Autodesk Inventor part; units mm, degrees
ref_plane "YZ Plane" through (0, 0, 0) normal (1, 0, 0) x (0, 1, 0)
ref_plane "XZ Plane" through (0, 0, 0) normal (0, 1, 0) x (-1, 0, 0)
ref_plane "XY Plane" through (0, 0, 0) normal (0, 0, 1) x (1, 0, 0)
sketch "スケッチ1" plane through (0, 0, 0) normal (0, 0, 1) x (1, 0, 0)
  line L0 (0, 0) -> (80, 0)
  line L1 (80, 0) -> (80, 60)
  line L2 (80, 60) -> (0, 60)
  line L3 (0, 60) -> (0, 0)
  dimension "d0" = 80
  dimension "d1" = 60
extrude "押し出し1" add sketch "スケッチ1" along normal blind 3
sketch "スケッチ2" plane through (0, 0, 3) normal (0, 0, 1) x (1, 0, 0)
  point P0 (0, 0)
sketch "スケッチ3" plane through (0, 0, 3) normal (0, 0, 1) x (1, 0, 0)
  line L0 (0, 0) -> (80, 0)
  line L1 (15, 0) -> (15, 60) construction
  line L2 (15, 0) -> (75, 0) construction
  line L3 (0, 60) -> (0, 0)
  circle A0 centre (7.5, 30) radius 1.6
  circle A1 centre (7.5, 40) radius 1.6
  circle A2 centre (7.5, 20) radius 1.6
  line L4 (80, 60) -> (0, 60)
  line L5 (40, 60) -> (40, 0) construction
  circle A3 centre (72.5, 30) radius 1.6
  circle A4 centre (72.5, 40) radius 1.6
  circle A5 centre (72.5, 20) radius 1.6
  point P0 (0, 30)
  dimension "d4" = 60
  dimension "d5" = 90
  dimension "d6" = 15
  dimension "d7" = 3.2
  dimension "d8" = 7.5
  dimension "d9" = 30
  dimension "d10" = 3.2
  dimension "d11" = 3.2
  dimension "d12" = 10
  dimension "d13" = 10
  dimension "d14" = 40
hole "穴1" at (7.5, 40, 3) at (7.5, 30, 3) at (7.5, 20, 3) at (72.5, 40, 3) at (72.5, 30, 3) at (72.5, 20, 3) direction (0, 0, -1) diameter 3.2 end through all
sketch "スケッチ4" plane through (0, 0, 3) normal (0, 0, 1) x (1, 0, 0)
  circle A0 centre (40, 30) radius 7.5
  line L0 (80, 60) -> (0, 60)
  line L1 (80, 0) -> (80, 60)
  point P0 (0, 0)
  dimension "d22" = 15
  dimension "d23" = 30
  dimension "d24" = 40
extrude "押し出し2" cut sketch "スケッチ4" against normal blind 3
sketch "スケッチ5" plane through (0, 0, 3) normal (0, 0, 1) x (1, 0, 0)
  point P0 (0, 0)
sketch "スケッチ6" plane through (0, 0, 3) normal (0, 0, 1) x (1, 0, 0)
  circle A0 centre (40, 30) radius 7.5
  circle A1 centre (40, 30) radius 12.05
  point P0 (0, 0)
  dimension "d27" = 24.1
extrude "押し出し3" cut sketch "スケッチ6" against normal blind 3
sketch "スケッチ7" plane through (0, 0, 3) normal (0, 0, 1) x (1, 0, 0)
  circle A0 centre (40, 30) radius 12.05
  line L0 (0, 0) -> (80, 0)
  point P0 (62.851, 30)
  point P1 (17.149, 30)
  dimension "d30" = 22.851
  dimension "d31" = 22.851
  dimension "d32" = 30
  dimension "d33" = 30
hole "穴2" at (17.149, 30, 3) at (62.851, 30, 3) direction (0, 0, -1) diameter 3.2 end through all
fillet "フィレット1" radius 6 4 edges at (0, 60, 1.5) (80, 60, 1.5) (80, 0, 1.5) (0, 0, 1.5)
sketch "スケッチ8" plane through (0, 0, 3) normal (0, 0, 1) x (1, 0, 0)
  point P0 (0, 0)
sketch "スケッチ9" plane through (0, 0, 3) normal (0, 0, 1) x (1, 0, 0)
  circle A0 centre (40, 30) radius 12.05
  circle A1 centre (40, 30) radius 9.6
  point P0 (0, 0)
  dimension "d42" = 19.2
extrude "押し出し4" add sketch "スケッチ9" against normal blind 3
properties part number "射出_エンコーダー固定2" material "アルミニウム 6061"
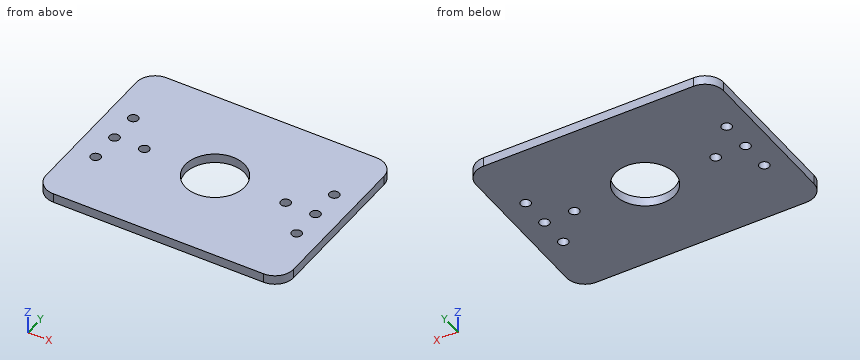
Read the model definition and answer for the solid it produces. Units are mm, in the model's axes. Coordinates: 2 decimals unless noted, no trailing zeros. Write each loop counter-clockwise with the first axis right and the second up, starting at its lowest first coordinate (ties: lowest second). Pieces come first, ordered by that corner, then holes. Notation, with made-up numbers: (2.25, 24.25) - (8.25, 24.25) arc R21 cw to (8.25, 33.25) - close; hole circle Ø6 at (7, 68.5). An arc over 180 degrees is marked (long way). One line per question, with ' | ' between items.
Q1. Find section D-D, the plane x = 34. Write down the section's boundary in (y, z), plus the area to 3 significant figures.
Result set:
outline: (0, 0) - (22.51, 0) - (22.51, 3) - (0, 3) - close; (37.49, 0) - (60, 0) - (60, 3) - (37.49, 3) - close | area: 135 mm^2
Q2. Consider L1, parallel to Y at x = 7.5, z = 2.15; L2, parallel to X at y = 40, z = 2.25; L3, parallel to Y at x = 8, z = 2.4. Determine where each line is inside the solid, lowest interval first. Write a range as [from, to].
Result set:
L1: [0, 18.4], [21.6, 28.4], [31.6, 38.4], [41.6, 60] | L2: [0, 5.9], [9.1, 70.9], [74.1, 80] | L3: [0, 18.48], [21.52, 28.48], [31.52, 38.48], [41.52, 60]
Q3. Find section C-C, the plane z = 0.6. State how many separate pieces and enclosed holes the cut face has, plus the area to 3 significant figures.
Result set:
separate pieces: 1 | enclosed holes: 9 | area: 4,420 mm^2
Q4. Find section A-A, the plane x = 7.5. Write down the section's boundary in (y, z).
Result set:
outline: (0, 0) - (18.4, 0) - (18.4, 3) - (0, 3) - close; (21.6, 0) - (28.4, 0) - (28.4, 3) - (21.6, 3) - close; (31.6, 0) - (38.4, 0) - (38.4, 3) - (31.6, 3) - close; (41.6, 0) - (60, 0) - (60, 3) - (41.6, 3) - close
Q5. Find section B-B, the plane x = 45. Write down the section's boundary in (y, z).
Result set:
outline: (0, 0) - (21.8, 0) - (21.8, 3) - (0, 3) - close; (38.2, 0) - (60, 0) - (60, 3) - (38.2, 3) - close
